Here's how the part is built. I have some questions about the finished solid (model axes, mm). Face numbers are marked on the shaded views. A direction names the side the tool comes from. Round coordinates to 2 decimals unless told otherwise and drop trailing zeros. Order: outer loops, then holes, each group sorted by start corner. A loop starts at its lowest first (then second) coordinate and runs counter-clockwise, first axis right, second up. Notation, with made-up numbers: M 43,14.5 L 69,14.5 A21 cw 69,34.5 Z; hole C 33.5,30.25 d6. An arc over 180 degrees is marked long. Answer as CSV lines item,"result". Start each with the question number.
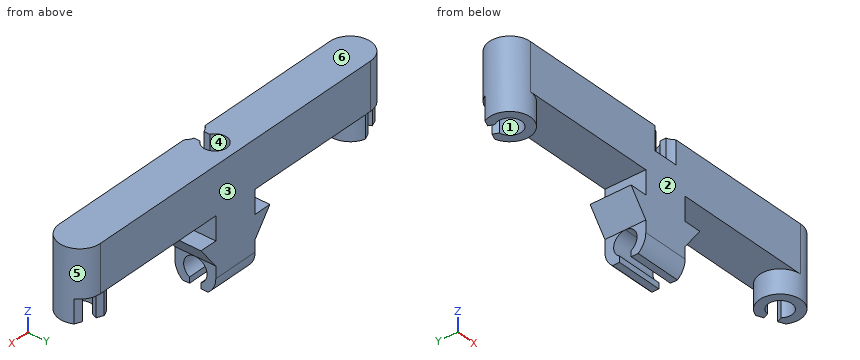
```python
from build123d import *

# Parameters (mm, degrees)
EXTRUDE_1_DEPTH     = 4
SKETCH_2_W          = 4
SKETCH_2_H          = 3.5
EXTRUDE_2_DEPTH     = 2
EXTRUDE_3_DEPTH     = 3.5
SKETCH_4_R          = 1.75
EXTRUDE_4_DEPTH     = 2
SKETCH_5_R          = 1.471524952
CUT_EXTRUDE_2_DEPTH = 2
SKETCH_7_W          = 4
SKETCH_7_H          = 3.5
EXTRUDE_5_DEPTH     = 4
CUT_EXTRUDE_4_DEPTH = 4
CUT_EXTRUDE_5_DEPTH = 2


with BuildPart() as part:
    # Sketch 1 → Extrude 1 (new body)
    with BuildSketch(Plane.XY):
        with BuildLine():
            Line((-13.7534088, 1.75), (13.7534088, 1.75))
            ThreePointArc((13.7534088, 1.75), (15.5034088, 0), (13.7534088, -1.75))
            Line((13.7534088, -1.75), (-13.7534088, -1.75))
            ThreePointArc((-13.7534088, -1.75), (-15.5034088, 0), (-13.7534088, 1.75))
        make_face()
    extrude(amount=EXTRUDE_1_DEPTH)

    # Sketch 2 → Extrude 2 (add)
    with BuildSketch(Plane(origin=(0, 0, 0), x_dir=(-1, 0, 0), z_dir=(0, 0, -1))):
        Rectangle(SKETCH_2_W, SKETCH_2_H)
    extrude(amount=EXTRUDE_2_DEPTH)

    # Sketch 3 → Extrude 3 (add)
    with BuildSketch(Plane(origin=(0, 1.75, 0), x_dir=(1, 0, 0), z_dir=(0, 1, 0))):
        Polygon((3.5, 2), (-3.5, 2), (-2, 4), (2, 4), align=None)
    extrude(amount=-EXTRUDE_3_DEPTH)

    # Sketch 4 → Extrude 4 (add)
    with BuildSketch(Plane(origin=(0, 0, 0), x_dir=(-1, 0, 0), z_dir=(0, 0, -1))):
        with Locations((-13.7534088, 0)):
            Circle(SKETCH_4_R)
        with Locations((13.7534088, 0)):
            Circle(SKETCH_4_R)
    extrude(amount=EXTRUDE_4_DEPTH)

    # Sketch 5 → Cut-Extrude 2 (cut)
    with BuildSketch(Plane.XY.offset(4)):
        with Locations((0, -2.75)):
            Circle(SKETCH_5_R)
        with BuildLine():
            Line((-0.5, -1.75), (-0.5, -0.866025404))
            ThreePointArc((-0.5, -0.866025404), (0, 1), (0.5, -0.866025404))
            Line((0.5, -0.866025404), (0.5, -1.75))
            Line((0.5, -1.75), (-0.5, -1.75))
        make_face()
    extrude(amount=-CUT_EXTRUDE_2_DEPTH, mode=Mode.SUBTRACT)

    # Sketch 7 → Extrude 5 (add)
    with BuildSketch(Plane(origin=(0, 0, -4), x_dir=(-1, 0, 0), z_dir=(0, 0, -1))):
        Rectangle(SKETCH_7_W, SKETCH_7_H)
    extrude(amount=EXTRUDE_5_DEPTH)

    # Sketch 8 → Cut-Extrude 4 (cut)
    with BuildSketch(Plane(origin=(2, 0, 0), x_dir=(0, 0, -1), z_dir=(1, 0, 0))):
        with BuildLine():
            Line((6.366025404, 1.093834812), (6.366025404, 0.5))
            Line((6.366025404, 0.5), (5.866025404, 0.5))
            ThreePointArc((5.866025404, 0.5), (4.741180961, 0.965925828), (4, 1.4e-08))
            ThreePointArc((4, 1.4e-08), (4.741180948, -0.965925825), (5.866025404, -0.5))
            Line((5.866025404, -0.5), (6.366025404, -0.5))
            Line((6.366025404, -0.5), (6.366025404, -1.093834812))
            ThreePointArc((6.366025404, -1.093834812), (5.75772326, -1.577452205), (5, -1.75))
            Line((5, -1.75), (8, -1.75))
            Line((8, -1.75), (8, 1.75))
            Line((8, 1.75), (5, 1.75))
            ThreePointArc((5, 1.75), (5.75772326, 1.577452205), (6.366025404, 1.093834812))
        make_face()
    extrude(amount=-CUT_EXTRUDE_4_DEPTH, mode=Mode.SUBTRACT)

    # Sketch 6 → Cut-Extrude 5 (cut)
    with BuildSketch(Plane(origin=(0, 0, -2), x_dir=(-1, 0, 0), z_dir=(0, 0, -1))):
        with BuildLine():
            Line((-14.756005706, 1.053956758), (-14.556907325, 0.595306745))
            ThreePointArc((-14.556907325, 0.595306745), (-13.355212038, -0.917300026), (-13.639607299, 0.993503507))
            Line((-13.639607299, 0.993503507), (-13.83870568, 1.45215352))
            Line((-13.83870568, 1.45215352), (-13.293980991, 1.68861662))
            ThreePointArc((-13.293980991, 1.68861662), (-13.625907559, 1.745349086), (-13.962555059, 1.737457292))
            ThreePointArc((-13.962555059, 1.737457292), (-14.450253134, 1.605275046), (-14.879855085, 1.33926053))
            ThreePointArc((-14.879855085, 1.33926053), (-15.115509691, 1.098717964), (-15.300730395, 0.817493658))
            Line((-15.300730395, 0.817493658), (-14.756005706, 1.053956758))
        make_face()
        with BuildLine():
            Line((13.83870568, 1.45215352), (13.639607299, 0.993503507))
            ThreePointArc((13.639607299, 0.993503507), (13.355212038, -0.917300026), (14.556907325, 0.595306745))
            Line((14.556907325, 0.595306745), (14.756005706, 1.053956758))
            Line((14.756005706, 1.053956758), (15.300730395, 0.817493658))
            ThreePointArc((15.300730395, 0.817493658), (15.115509691, 1.098717964), (14.879855085, 1.33926053))
            ThreePointArc((14.879855085, 1.33926053), (14.450253134, 1.605275046), (13.962555059, 1.737457292))
            ThreePointArc((13.962555059, 1.737457292), (13.625907559, 1.745349086), (13.293980991, 1.68861662))
            Line((13.293980991, 1.68861662), (13.83870568, 1.45215352))
        make_face()
    extrude(amount=-CUT_EXTRUDE_5_DEPTH, mode=Mode.SUBTRACT)


solid = part.part
```
Item 1: Which directions (+Z, -Z, +X, -X, +Y, -Y) give clear straight access to the entire face, cutting with the end or side of a thin tool? Please do the marked faces 4, 5 and 6.
Item 2: If I drill on line 1 along X through (y, z) = (0, -0.7); line 2 along X through (y, z) = (0, 3.6); line 3 along X through (y, z) = (0.75, -1.75), over which ranges is the centre line in solid material (lowest first)?
Item 3: For P1, Ø1.8, axis at x = 9, y = -0.5, coming from the -Z side; P2, Ø0.9, axis at y = -0.5, z = -4.5, coming from the -X side; P3, Ø0.9, axis at y = -0.5, z = -5.5, coming from the +X side, each with a flat end and sliding along its axis, tell me the tip position at first contact or that it passes through.
Item 4: We'd pull the mould along Y, two halves only. Please class the marked faces 1, 2 and 3: pulls with the +Y half, pulls with the -Y half, needs draft (parallel to the pull), parting line crosses it, or undercut.
Item 5: If we section it at D-D on z = -2.75: Please give me the cut outline in (x, y).
Item 6: If we section it at B-B on x = 0: Please give me the cut outline in (y, z).
Item 7: If we section it at C-C on x = -11.5: Please give me the cut outline in (y, z).
Item 8: If we section it at A-A on z = 2.75: Please give me the cut outline in (x, y).
Geometry says:
1,face 4,"+Z"
1,face 5,"-Z"
1,face 6,"+Z, +X, -X, +Y, -Y"
2,line 1,"-15.5 to -14.75, -12.75 to -12, -2 to 2, 12 to 12.75, 14.75 to 15.5"
2,line 2,"-15.5 to -1, 1 to 15.5"
2,line 3,"-15.33 to -14.62, -13.09 to -12.17, -2 to 2, 12.17 to 13.09, 14.62 to 15.33"
3,P1,"z = 0"
3,P2,"x = -2"
3,P3,"x = 2"
4,face 1,"undercut"
4,face 2,"pulls with the -Y half"
4,face 3,"pulls with the +Y half"
5,outline,"M -2.94,-1.75 L 2.94,-1.75 L 2.94,1.75 L -2.94,1.75 Z"
6,outline,"M -1.75,-5 A1.75 ccw -1.09,-6.37 L -0.5,-6.37 L -0.5,-5.87 A1 cw long 0.5,-5.87 L 0.5,-6.37 L 1.09,-6.37 A1.75 ccw 1.75,-5 L 1.75,4 L 1,4 L 1,2 L -1.75,2 Z"
7,outline,"M -1.75,0 L 1.75,0 L 1.75,4 L -1.75,4 Z"
8,outline,"M -13.75,-1.75 L -1.08,-1.75 A1.47 cw -0.5,-1.37 L -0.5,-0.87 A1 cw long 0.5,-0.87 L 0.5,-1.37 A1.47 cw 1.08,-1.75 L 13.75,-1.75 A1.75 ccw 13.75,1.75 L -13.75,1.75 A1.75 ccw Z"
